Geometry check sheet. Reference: the model listing, model coordinates, mm. Give positions to 0.01 mm unless a question says otherwise; leave off trailing zeros. Loops run counter-clockwise (first coordinate to the right, second up) from the corner with the lowest first, then second, coordinate; pieces in that order, holes last.
1. Go/stop test with flat-tipped pins: pin 1 Ø0.5 at (x, z) = (1, -30.5) entering from -Y; pin 2 Ø0.5 at (x, y) = (0.5, 4.5) entering from +Z. Record where each tip stops, or that it passes through.
2. Material ranges on L1, parallel to Z at x = 0.85, y = 0 (3 decimals); L2, parallel to Y at x = 0.35, z = 65; L3, parallel to Y at x = 1.35, z = -29, recorded low to high.
3. Cross-section at C-C, the plane x = 1. State how many separate pieces and enclosed holes the cut face has, plus the area to 3 significant figures.
4. Cross-section at D-D, the plane z = 57.5. Record the cut outline in (x, y), plus the area to 3 significant figures.
5. Cross-section at A-A, the plane y = 26.5. Record the cut outline in (x, z), plus the area to 3 significant figures.
6. Cross-section at B-B, the plane z = -30.5. Record the cut outline in (x, y).
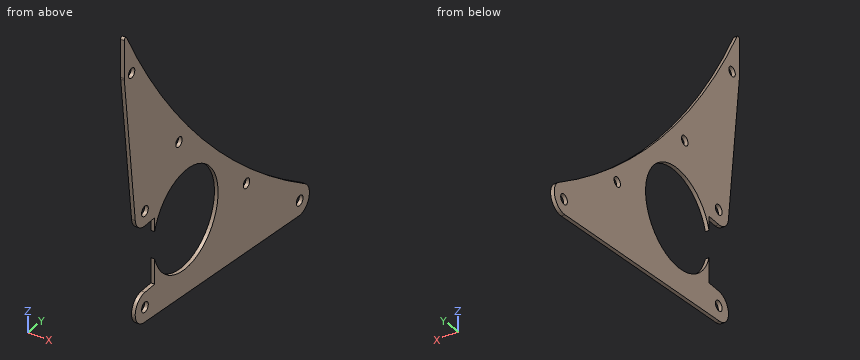
Autodesk Inventor part; units mm, degrees
ref_plane "YZ Plane" through (0, 0, 0) normal (1, 0, 0) x (0, 1, 0)
ref_plane "XZ Plane" through (0, 0, 0) normal (0, 1, 0) x (-1, 0, 0)
ref_plane "XY Plane" through (0, 0, 0) normal (0, 0, 1) x (1, 0, 0)
sketch "main" plane through (0, 0, 0) normal (0, 0, 1) x (1, 0, 0)
  circle A0 centre (-198.1135, 49.9495) radius 2.1844
  circle A1 centre (-97.0008, -1.1659) radius 2.1
  arc A2 (-97.6159, -7.486) -> (-93.6005, 4.197) centre (-97.0008, -1.1659) ccw
  arc A3 (-204.4247, 49.249) -> (-198.1135, 43.5995) centre (-198.1135, 49.9495) ccw
  arc A4 (-210.0929, 131.0519) -> (-93.6005, 4.197) centre (83.8489, 284.0666) ccw
  circle A5 centre (-206.8262, 114.0524) radius 2.0828
  arc A6 (-210.0929, 131.0519) -> (-211.5759, 130.5326) centre (-210.797, 130.6854) ccw
  circle A7 centre (-131.7625, 25.4) radius 2.0828
  line L0 (-198.7286, 2.3544) -> (-97.6159, -7.486)
  circle A8 centre (-198.1135, 8.6745) radius 2.1848
  arc A9 (-198.1135, 15.0245) -> (-198.7286, 2.3544) centre (-198.1135, 8.6745) ccw
  line L1 (-211.5828, 130.7972) -> (-211.5828, 113.8158)
  arc A10 (-211.5828, 114.289) -> (-211.5596, 113.527) centre (-206.8262, 114.0524) ccw
  line L2 (-211.5596, 113.527) -> (-204.4247, 49.249)
  circle A11 centre (-175.8885, 67.412) radius 2.0955
  arc A12 (-191.7635, 25.8768) -> (-191.7635, 37.6232) centre (-171.45, 31.75) ccw
  line L3 (-191.7635, 43.5995) -> (-191.7635, 37.6232)
  line L4 (-191.7635, 15.0245) -> (-191.7635, 25.8768)
  point P0 (1.1251, 9.7944)
  point P1 (-211.9386, 134.6509)
  point P2 (-191.7635, 49.9495)
  dimension "d7" = 12.7
  dimension "d8" = 4.1656
  dimension "d9" = 6.35
  dimension "d13" = 4.1656
  dimension "d20" = 0
  dimension "d21" = 6.35
  dimension "d26" = 9.525
  dimension "d27" = 4.191
  dimension "d29" = 42.291
sketch "Sketch1" plane through (0, 0, 0) normal (1, 0, 0) x (0, 1, 0)
  line L0 (6.35, -9.525) -> (6.35, -7.9375)
  line L1 (0, -6.35) -> (6.35, -6.35)
  line L2 (0, -34.925) -> (6.35, -34.925)
  circle A0 centre (101.1127, -51.1154) radius 2.1844
  circle A1 centre (0, 0) radius 2.1844
  circle A2 centre (101.1127, -51.1154) radius 2.1
  arc A3 (100.4976, -57.4355) -> (104.5129, -45.7525) centre (101.1127, -51.1154) ccw
  arc A4 (-6.3112, -0.7006) -> (0, -6.35) centre (0, 0) ccw
  arc A5 (-11.9794, 81.1024) -> (104.5129, -45.7525) centre (281.9624, 234.117) ccw
  circle A6 centre (-8.7127, 64.1028) radius 2.0828
  arc A7 (-11.9794, 81.1024) -> (-13.4624, 80.5831) centre (-12.6835, 80.7359) ccw
  circle A8 centre (66.351, -24.5495) radius 2.0828
  line L3 (-0.6151, -47.5951) -> (100.4976, -57.4355)
  circle A9 centre (0, -41.275) radius 2.1848
  arc A10 (0, -34.925) -> (-0.6151, -47.5951) centre (0, -41.275) ccw
  line L4 (-13.4693, 80.8476) -> (-13.4693, 63.8663)
  arc A11 (-13.4693, 64.3394) -> (-13.4461, 63.5774) centre (-8.7127, 64.1028) ccw
  line L5 (-13.4461, 63.5774) -> (-6.3112, -0.7006)
  circle A12 centre (22.225, 17.4625) radius 2.0955
  arc A13 (6.35, -24.0727) -> (6.35, -12.3264) centre (26.6635, -18.1995) ccw
  line L6 (6.35, -6.35) -> (6.35, -12.3264)
  line L7 (6.35, -34.925) -> (6.35, -24.0727)
  point P0 (0, -6.35)
  point P1 (0, -34.925)
  point P2 (-13.4693, 80.6241)
  point P3 (6.35, -6.35)
  point P4 (6.35, -34.925)
extrude "Extrusion1" add sketch "Sketch1" along normal blind 1.5875 contours L0 L6 L1 A4 L5 A11 L4 A7 A5 A3 L3 A10 L2 L7 A13 | A11 L4 | A7 L4
equation "\"BendRadius\" = Thickness"
equation "\"BendReliefWidth\" = Thickness"
equation "\"BendReliefDepth\" = 0.5 * Thickness"
equation "\"CornerReliefSize\" = 4 * Thickness"
equation "\"MinimumRemnant\" = 2 * Thickness"
equation "\"TransitionRadius\" = BendRadius"
equation "\"JacobiRadiusSize\" = BendRadius"
equation "\"GapSize\" = Thickness"
properties part number "Ramp V2" material "Acetal Resin, White"
Result:
1. pin 1: stops at y = 6.35
1. pin 2: stops at z = 53.31
2. L1: z = -47.655 to -43.46, -39.09 to -34.925, -6.35 to -2.184, 2.184 to 60.012
2. L2: y = -13.47 to -10.59, -6.83 to -3.02
2. L3: y = 6.35 to 8.48, 44.84 to 80.51
3. separate pieces: 1
3. enclosed holes: 6
3. area: 4,600 mm2
4. outline: (0, -12.77) - (1.59, -12.77) - (1.59, 1.57) - (0, 1.57) - close
4. area: 22.8 mm2
5. outline: (0, -50.23) - (1.59, -50.23) - (1.59, -39.34) - (0, -39.34) - close; (0, 2.95) - (1.59, 2.95) - (1.59, 23.04) - (0, 23.04) - close
5. area: 49.2 mm2
6. outline: (0, 6.35) - (1.59, 6.35) - (1.59, 9.46) - (0, 9.46) - close; (0, 43.86) - (1.59, 43.86) - (1.59, 82.48) - (0, 82.48) - close
